Can you work these out from the model? Positions are in its coordinate system, mm. Face numbers are marked on the shaded views. Coordinates: 2 decimals unless noted, no trailing zeros. Order: outer loops, then holes, each group sorted by start corner. A loop starts at its lowest first (then second) coordinate and runs counter-clockwise, first axis right, second up. Notation, with made-up numbers: (-2, 65.5) -> (33, 65.5) arc R14 cw to (33, 72.5) -> close; hole circle Ø4 at (-31, 58.25). An arc over 180 degrees is marked (long way). Answer as a JSON object with one key per item and string values. Group by question number.
(1) I want a section at A-A, the plane x = 0. List the corners of the cut face in (y, z) for me.
(2) I want a section at D-D, the plane x = -29.5. List the corners of the cut face in (y, z) for me, plus the area to 3 significant figures.
(3) I want a section at B-B, the plane z = 0. List the corners of the cut face in (x, y) for me, plus the area to 3 significant figures.
(4) If we mould it in two halves opening along Z, with no side actions, what happens to the marked faces 1, 2 and 3? For each: pulls with the +Z half, pulls with the -Z half, needs draft (parallel to the pull), parting line crosses it, or undercut.
(5) I need wall thicknesses on line 1 (Z direction, x = 0, y = 6.9); line 2 (Z direction, x = 0, y = 8.25); line 3 (Y direction, x = -25.5, z = -7). Which ranges of each line are inside material? Lowest first, please.
(6) For pin 1 (1 mm diameter, centred on x = 12.5, z = -26.5, fed in from +Y); pin 2 (2 mm diameter, centred on y = 6.5, z = -12, fed in from -X); pin 3 (4 mm diameter, centred on y = 8, z = 27, fed in from +X) (3 decimals), each with a flat end and sliding along its axis, tell me the tip position at first contact or that it passes through.
(7) I want a section at C-C, the plane z = -30. List the corners of the cut face in (x, y) for me, plus the area to 3 significant figures.
Autodesk Inventor part; units mm, degrees
ref_plane "YZ Plane" through (0, 0, 0) normal (1, 0, 0) x (0, 1, 0)
ref_plane "XZ Plane" through (0, 0, 0) normal (0, 1, 0) x (-1, 0, 0)
ref_plane "XY Plane" through (0, 0, 0) normal (0, 0, 1) x (1, 0, 0)
sketch "Эскиз1" plane through (0, 0, 0) normal (0, 1, 0) x (-1, 0, 0)
  point P0 (0, 0)
sketch "Эскиз2" plane through (0, 0, 0) normal (0, 1, 0) x (-1, 0, 0)
  circle A0 centre (0, 0) radius 40
  dimension "d0" = 80
extrude "Выдавливание1" add sketch "Эскиз2" along normal blind 8
sketch "Эскиз3" plane through (0, 0, 0) normal (0, -1, 0) x (1, 0, 0)
  circle A0 centre (0, 30) radius 8.2
  circle A1 centre (0, -30) radius 8.2
  point P0 (0, 0)
  dimension "d3" = 16.4
  dimension "d4" = 16.4
sketch "Эскиз4" plane through (0, 0, 0) normal (1, 0, 0) x (0, 1, 0)
  line L0 (0, 40) -> (0, -40)
  line L1 (0, 29.8473) -> (0, 38.0473)
  line L2 (0, 38.0473) -> (8.2, 29.8473)
  line L3 (8.2, 29.8473) -> (0, 29.8473)
  point P0 (0, 0)
  dimension "d5" = 8.2
  dimension "d6" = 45
revolve "Вращение1" cut sketch "Эскиз4" angle 360 about axis through (0, 8.2, 29.8473) along (0, -1, 0)
sketch "Эскиз5" plane through (0, 0, 0) normal (1, 0, 0) x (0, 1, 0)
  point P0 (0, 0)
sketch "Эскиз6" plane through (0, 0, 0) normal (1, 0, 0) x (0, 1, 0)
  line L0 (0, 40) -> (0, -40)
  line L1 (0, -30) -> (0, -38.2)
  line L2 (0, -38.2) -> (8.2, -30)
  line L3 (8.2, -30) -> (0, -30)
  point P0 (0, 0)
  dimension "d8" = 8.2
  dimension "d9" = 45
revolve "Вращение2" cut sketch "Эскиз6" angle 360 about axis through (0, 8.2, -30) along (0, -1, 0)
sketch "Эскиз7" plane through (0, 8, 0) normal (0, 1, 0) x (1, 0, 0)
  circle A0 centre (0, 30) radius 0.2
  circle A1 centre (0, -29.8473) radius 0.2
  point P0 (0, 0)
hole "Отверстие1" at (0, 8, -30) at (0, 8, 29.8473) direction (0, -1, 0) diameter 9 end through all
sketch "Эскиз8" plane through (0, 8, 0) normal (0, 1, 0) x (1, 0, 0)
  circle A0 centre (0, 0) radius 22
  dimension "d18" = 44
extrude "Выдавливание2" add sketch "Эскиз8" along normal blind 6
sketch "Эскиз9" plane through (0, 14, 0) normal (0, 1, 0) x (1, 0, 0)
  point P0 (0, 0)
  point P1 (0, 0)
hole "Отверстие2" at (0, 14, 0) direction (0, -1, 0) diameter 32 end through all
chamfer "Фаска1" distance 2 angle 45 1 edges at (-22, 14, 0)
properties part number "крышка"
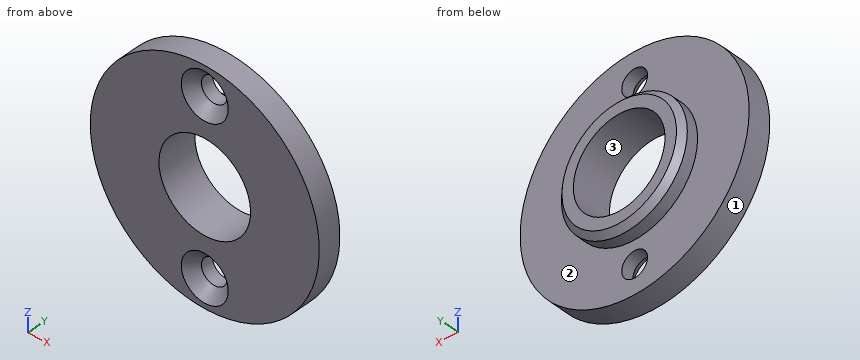
Computed values:
{
 "1": {"outline": "(0, -40) -> (8, -40) -> (8, -34.5) -> (3.7, -34.5) -> (0, -38.2) -> close; (0, -21.8) -> (3.7, -25.5) -> (8, -25.5) -> (8, -22) -> (12, -22) -> (14, -20) -> (14, -16) -> (0, -16) -> close; (0, 16) -> (14, 16) -> (14, 20) -> (12, 22) -> (8, 22) -> (8, 25.35) -> (3.7, 25.35) -> (0, 21.65) -> close; (0, 38.05) -> (3.7, 34.35) -> (8, 34.35) -> (8, 40) -> (0, 40) -> close"},
 "2": {"outline": "(0, -27.01) -> (8, -27.01) -> (8, 27.01) -> (0, 27.01) -> close", "area": "432 mm2"},
 "3": {"outline": "(-40, 0) -> (-16, 0) -> (-16, 14) -> (-20, 14) -> (-22, 12) -> (-22, 8) -> (-40, 8) -> close; (16, 0) -> (40, 0) -> (40, 8) -> (22, 8) -> (22, 12) -> (20, 14) -> (16, 14) -> close", "area": "452 mm2"},
 "4": {"face 1": "parting line crosses it", "face 2": "needs draft", "face 3": "undercut"},
 "5": {"line 1": "z = -40 to -34.5, -25.5 to -16, 16 to 25.35, 34.35 to 40", "line 2": "z = -22 to -16, 16 to 22", "line 3": "y = 0 to 8"},
 "6": {"pin 1": "stops at y = 8", "pin 2": "stops at x = -38.46", "pin 3": "stops at x = 31.225"},
 "7": {"outline": "(-26.46, 0) -> (-8.2, 0) -> (-4.5, 3.7) -> (-4.5, 8) -> (-26.46, 8) -> close; (4.5, 3.7) -> (8.2, 0) -> (26.46, 0) -> (26.46, 8) -> (4.5, 8) -> close", "area": "338 mm2"}
}
